Check sheet for the drawn part. Datum: minimum x, y, z corner. Units: mm. Give positions to 0.01 mm unless a question says otherwise; leave off trailing zeros. Loops run counter-clockwise (first coordinate to the right, second up) from the corner with the lowest first, then second, coordinate; pieces in that order, holes last. Notation, with made-up numbers: (-36.5, 67) - (13.5, 67) arc R17 cw to (13.5, 72) - close; hole circle Ø11 at (30, 23). An arc over 180 degrees is marked (long way). One line per item, written item: value. Start each with the question number.
1. Sectioned sample at D-D (x = 13.5). Record the cut outline in (y, z).
2. Mould release check, pull along Z, two halves, no side actions. Record for the marked faces 1, 2 and 3: pulls with the +Z half, pulls with the -Z half, needs draft (parallel to the pull), parting line crosses it, or undercut.
3. Scan lines: L1, parallel to Z at x = 29.21, y = 5 (3 decimals); L2, parallel to Z at x = 44.45, y = 14.5; L3, parallel to Z at x = 67.5, y = 7.5. Record each from-to range of solid material in increasing order. Write a range as [from, to].
4. Sectioned sample at C-C (y = 13). Record the cut outline in (x, z).
5. Gauge pin test, flat ends, axial feed: pin 1 (11.5 mm diameter, centred on x = 29.21, z = 59.69, fed in from +Y); pin 2 (1 mm diameter, centred on y = 3.5, z = 32.5, fed in from -X); pin 3 (5.5 mm diameter, centred on x = 44.45, z = 44.45, fed in from +Y); pin 4 (5 mm diameter, centred on x = 30, y = 5, fed in from +Z). Record the tip position at first contact, or that the pin passes through.
6. Sectioned sample at A-A (z = 59.69). Record the cut outline in (x, y) (3 decimals).
7. Sectioned sample at B-B (x = 45). Record the cut outline in (y, z).
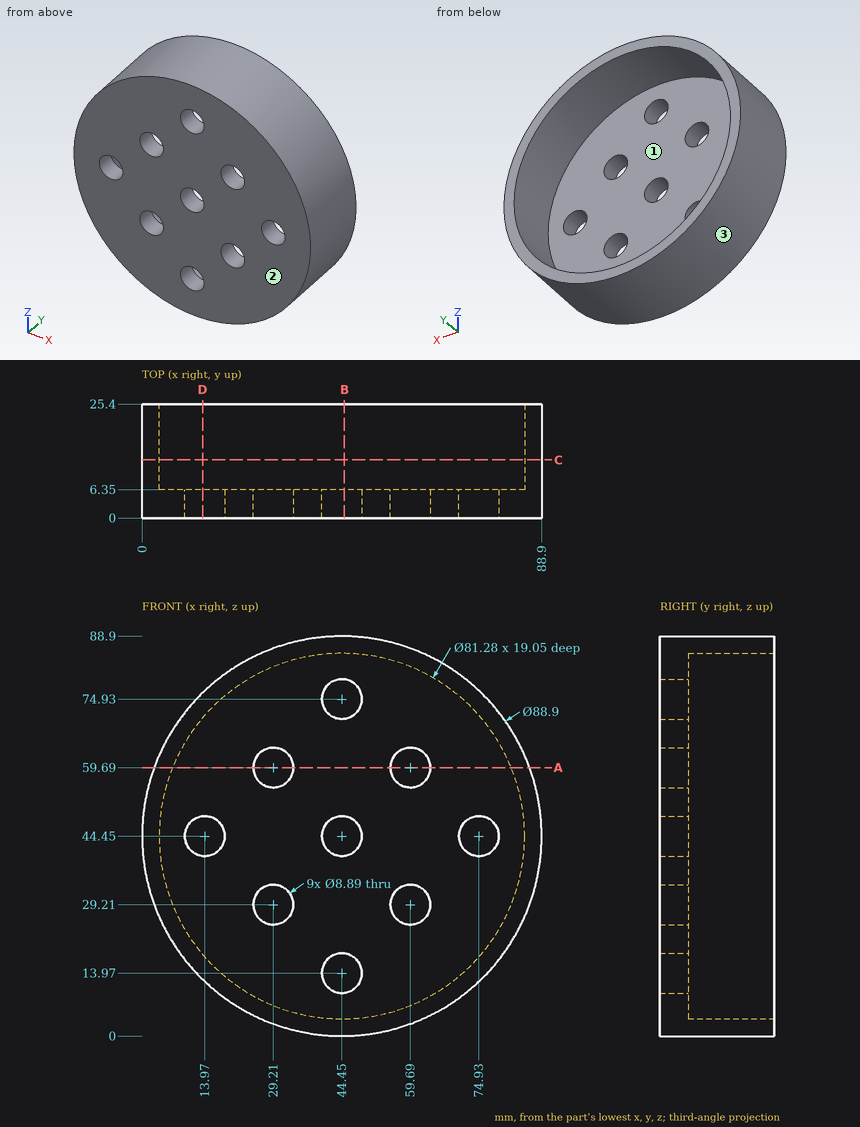
Results are:
1. outline: (0, 12.55) - (25.4, 12.55) - (25.4, 18.11) - (6.35, 18.11) - (6.35, 40.03) - (0, 40.03) - close; (0, 48.87) - (6.35, 48.87) - (6.35, 70.79) - (25.4, 70.79) - (25.4, 76.35) - (0, 76.35) - close
2. face 1: undercut
2. face 2: needs draft
2. face 3: parting line crosses it
3. L1: z = [2.694, 24.765], [33.655, 55.245], [64.135, 86.206]
3. L2: z = [0, 3.81], [85.09, 88.9]
3. L3: z = [6.44, 10.98], [77.92, 82.46]
4. outline: circle Ø88.9 at (44.45, 44.45); hole circle Ø81.28 at (44.45, 44.45)
5. pin 1: stops at y = 6.35
5. pin 2: stops at x = 1.5
5. pin 3: passes through
5. pin 4: stops at z = 87.26
6. outline: (2.694, 0) - (24.765, 0) - (24.765, 6.35) - (6.776, 6.35) - (6.776, 25.4) - (2.694, 25.4) - close; (33.655, 0) - (55.245, 0) - (55.245, 6.35) - (33.655, 6.35) - close; (64.135, 0) - (86.206, 0) - (86.206, 25.4) - (82.124, 25.4) - (82.124, 6.35) - (64.135, 6.35) - close
7. outline: (0, 0) - (25.4, 0) - (25.4, 3.81) - (6.35, 3.81) - (6.35, 9.56) - (0, 9.56) - close; (0, 18.38) - (6.35, 18.38) - (6.35, 40.04) - (0, 40.04) - close; (0, 48.86) - (6.35, 48.86) - (6.35, 70.52) - (0, 70.52) - close; (0, 79.34) - (6.35, 79.34) - (6.35, 85.09) - (25.4, 85.09) - (25.4, 88.9) - (0, 88.9) - close
